from build123d import *

# Parameters (mm, degrees)
SKETCH_1_W          = 95
SKETCH_1_H          = 40
SKETCH_1_R          = 2.025
EXTRUDE_1_DEPTH     = 4
FILLET_1_R          = 4.5
SKETCH_2_W          = 79
SKETCH_2_H          = 24
CUT_EXTRUDE_1_DEPTH = 10
FILLET_2_R          = 3
SKETCH_3_R          = 2.025
CUT_EXTRUDE_2_DEPTH = 10
SKETCH_4_R          = 6
SKETCH_4_R_2        = 2.025
EXTRUDE_2_DEPTH     = 4
FILLET_3_R          = 5


with BuildPart() as part:
    # 草图1 → 凸台-拉伸1 (new body)
    with BuildSketch(Plane.XY):
        Rectangle(SKETCH_1_W, SKETCH_1_H)
        with Locations((-42, -14.5)):
            Circle(SKETCH_1_R, mode=Mode.SUBTRACT)
        with Locations((42, -14.5)):
            Circle(SKETCH_1_R, mode=Mode.SUBTRACT)
        with Locations((42, 14.5)):
            Circle(SKETCH_1_R, mode=Mode.SUBTRACT)
        with Locations((-42, 14.5)):
            Circle(SKETCH_1_R, mode=Mode.SUBTRACT)
        with BuildLine():
            Line((47.5, -20), (-47.5, -20))
            Line((-47.5, -20), (-47.5, -25))
            Line((-47.5, -25), (-117.089181798, -94.947092696))
            ThreePointArc((-117.089181798, -94.947092696), (-113.838679914, -92.766120181), (-110, -92))
            Line((-110, -92), (110, -92))
            ThreePointArc((110, -92), (113.838679914, -92.766120181), (117.089181798, -94.947092696))
            Line((117.089181798, -94.947092696), (47.5, -25))
            Line((47.5, -25), (47.5, -20))
        make_face()
        with BuildLine():
            Line((110, -92), (-110, -92))
            ThreePointArc((-110, -92), (-120, -102), (-110, -112))
            Line((-110, -112), (110, -112))
            ThreePointArc((110, -112), (120, -102), (110, -92))
        make_face()
        with Locations((110, -102)):
            Circle(SKETCH_1_R, mode=Mode.SUBTRACT)
        with Locations((55, -102)):
            Circle(SKETCH_1_R, mode=Mode.SUBTRACT)
        with Locations((0, -102)):
            Circle(SKETCH_1_R, mode=Mode.SUBTRACT)
        with Locations((-55, -102)):
            Circle(SKETCH_1_R, mode=Mode.SUBTRACT)
        with Locations((-110, -102)):
            Circle(SKETCH_1_R, mode=Mode.SUBTRACT)
    extrude(amount=EXTRUDE_1_DEPTH)

    # 圆角1
    fillet_1_edges = [part.edges().sort_by_distance(p)[0] for p in [
        (-47.5, -25, 2),
        (-47.5, 20, 2),
        (47.5, 20, 2),
        (47.5, -25, 2),
    ]]
    fillet(fillet_1_edges, radius=FILLET_1_R)

    # 草图2 → 切除-拉伸1 (cut)
    with BuildSketch(Plane.XY.offset(4)):
        Rectangle(SKETCH_2_W, SKETCH_2_H)
        Polygon((-39.5, -84.228054643), (-39.5, -20), (-4, -20), (-4, -55), align=None)
        Polygon((4, -55), (39.5, -84.228054643), (39.5, -20), (4, -20), align=None)
        Polygon((39.5, -92), (0, -59.478643425), (0, -92), align=None)
        Polygon((0, -92), (0, -59.478643425), (-39.5, -92), align=None)
        Polygon((51.5, -92), (51.5, -38.945557904), (104.282968869, -92), align=None)
        Polygon((-104.282968869, -92), (-51.5, -92), (-51.5, -38.945557904), align=None)
        with BuildLine():
            Line((-100, -106), (-65, -106))
            ThreePointArc((-65, -106), (-61, -102), (-65, -98))
            Line((-65, -98), (-100, -98))
            ThreePointArc((-100, -98), (-104, -102), (-100, -106))
        make_face()
        with BuildLine():
            Line((-45, -106), (-10, -106))
            ThreePointArc((-10, -106), (-6, -102), (-10, -98))
            Line((-10, -98), (-45, -98))
            ThreePointArc((-45, -98), (-49, -102), (-45, -106))
        make_face()
        with BuildLine():
            Line((10, -106), (45, -106))
            ThreePointArc((45, -106), (49, -102), (45, -98))
            Line((45, -98), (10, -98))
            ThreePointArc((10, -98), (6, -102), (10, -106))
        make_face()
        with BuildLine():
            Line((65, -106), (100, -106))
            ThreePointArc((100, -106), (104, -102), (100, -98))
            Line((100, -98), (65, -98))
            ThreePointArc((65, -98), (61, -102), (65, -106))
        make_face()
    extrude(amount=-CUT_EXTRUDE_1_DEPTH, mode=Mode.SUBTRACT)

    # 圆角2
    fillet_2_edges = [part.edges().sort_by_distance(p)[0] for p in [
        (39.5, -12, 2),
        (-39.5, -12, 2),
        (-39.5, 12, 2),
        (39.5, 12, 2),
        (51.5, -92, 2),
        (51.5, -38.945557904, 2),
        (104.282968869, -92, 2),
        (0, -59.478643425, 2),
        (39.5, -92, 2),
        (-39.5, -92, 2),
        (39.5, -84.228054643, 2),
        (4, -55, 2),
        (4, -20, 2),
        (39.5, -20, 2),
        (-39.5, -84.228054643, 2),
        (-39.5, -20, 2),
        (-4, -20, 2),
        (-4, -55, 2),
        (-51.5, -92, 2),
        (-104.282968869, -92, 2),
        (-51.5, -38.945557904, 2),
    ]]
    fillet(fillet_2_edges, radius=FILLET_2_R)

    # 草图3 → 切除-拉伸2 (cut)
    with BuildSketch(Plane.XY.offset(4)):
        with Locations((-47.5, -34.5)):
            Circle(SKETCH_3_R)
        with Locations((-47.5, -59.5)):
            Circle(SKETCH_3_R)
        with Locations((47.5, -34.5)):
            Circle(SKETCH_3_R)
        with Locations((47.5, -59.5)):
            Circle(SKETCH_3_R)
    extrude(amount=-CUT_EXTRUDE_2_DEPTH, mode=Mode.SUBTRACT)

    # 草图4 → 凸台-拉伸2 (add)
    with BuildSketch(Plane.XY.offset(4)):
        with Locations((-47.5, -59.5)):
            Circle(SKETCH_4_R)
        with Locations((-47.5, -59.5)):
            Circle(SKETCH_4_R_2, mode=Mode.SUBTRACT)
        with Locations((47.5, -59.5)):
            Circle(SKETCH_4_R)
        with Locations((47.5, -59.5)):
            Circle(SKETCH_4_R_2, mode=Mode.SUBTRACT)
    extrude(amount=-EXTRUDE_2_DEPTH)

    # 圆角3
    fillet_3_edges = [part.edges().sort_by_distance(p)[0] for p in [
        (-51.5, -63.972135955, 2),
        (-51.5, -55.027864045, 2),
        (51.5, -63.972135955, 2),
        (51.5, -55.027864045, 2),
    ]]
    fillet(fillet_3_edges, radius=FILLET_3_R)


solid = part.part
Part model, mm, in its own coordinate system. A direction names the side the tool comes from. Round coordinates to 2 decimals unless told otherwise and drop trailing zeros. Write each loop counter-clockwise with the first axis right and the second up, starting at its lowest first coordinate (ties: lowest second). Pieces come first, ordered by that corner, then holes. Notation, with made-up numbers: M 19,-31 L 30,-31 A17 cw 30,-17 Z; hole C 47.5,68.5 d2. An arc over 180 degrees is marked long. Return JSON: item names as keys, results as strings. Group by question number.
(1) Two-plate mould, pull along X, no slides. Class faces 3 (the face through (-46.217, 18.647, 2.028)), 4 (the face through (-1, -55, 4)), 5 (the face through (-77.61, -65.19, 2.03)), 6 (the face through (-17.26, -73.69, 2.03)): +X half, -X half, draft (parallel to the pull), parting line (faces both ways), or undercut.
(2) Saw through at A-A on y = 1. Write the cut outline in (x, z), then the cut area to 3 significant figures.
(3) Which spindle directions (+Z, -Z, +X, -X, +Y, -Y) get a long thin tool onto all of the face, cutting with end or side? Do faces 1 (the face through (19.637, -67.874, 2.028)), 2 (the face through (-82.47, -60.15, 1.97)). Say none if no direction does.
(4) Saw through at C-C on z = 2.9. Count the separate pieces of the cut face and the enclosed holes in it, then the cut area to 3 significant figures.
(5) Pin check, flat tips, straight feed: pin 1 Ø2 at (x, z) = (75, 3) entering from +Y; pin 2 Ø1.2 at (y, z) = (-4.5, 2.5) entering from -X; pin 3 Ø2 at (y, z) = (-51, 1.5) entering from +X. Stop position of each tip, or through.
(6) Drill centre lines: probe 1 along Y at (x, z) = (-42, 0.8) (3 decimals); probe 2 along Y at (x, z) = (0, 0.9) (3 decimals); probe 3 along Y at (x, z) = (-66, 1.8). Where is each one in solid material? Low to high.
(7) Saw through at B-B on x = -25. Write the cut outline in (y, z).
(8) Saw through at D-D on y = -69. Write the cut outline in (x, z), then the cut area to 3 significant figures.
Returned:
{
 "1": {"face 3": "-X half", "face 4": "draft", "face 5": "undercut", "face 6": "undercut"},
 "2": {"outline": "M -47.5,0 L -39.5,0 L -39.5,4 L -47.5,4 Z; M 39.5,0 L 47.5,0 L 47.5,4 L 39.5,4 Z", "area": "64.0 mm²"},
 "3": {"face 1": "+Z, -Z", "face 2": "+Z, -Z, -X, +Y"},
 "4": {"separate pieces": "1", "enclosed holes": "23", "area": "8,960 mm²"},
 "5": {"pin 1": "y = -51.64", "pin 2": "x = -47.5", "pin 3": "x = 74.36"},
 "6": {"probe 1": "-112 to -106, -98 to -16.525, -12.475 to 12.475, 16.525 to 20", "probe 2": "-112 to -104.025, -99.975 to -92, -60.365 to -12, 12 to 20", "probe 3": "-112 to -106, -98 to -92, -53.52 to -43.6"},
 "7": {"outline": "M -112,0 L -106,0 L -106,4 L -112,4 Z; M -98,0 L -92,0 L -92,4 L -98,4 Z; M -80.06,0 L -72.29,0 L -72.29,4 L -80.06,4 Z; M -20,0 L -12,0 L -12,4 L -20,4 Z; M 12,0 L 20,0 L 20,4 L 12,4 Z"},
 "8": {"outline": "M -91.27,0 L -81.4,0 L -81.4,4 L -91.27,4 Z; M -51.5,0 L -39.5,0 L -39.5,4 L -51.5,4 Z; M -21,0 L -11.56,0 L -11.56,4 L -21,4 Z; M 11.56,0 L 21,0 L 21,4 L 11.56,4 Z; M 39.5,0 L 51.5,0 L 51.5,4 L 39.5,4 Z; M 81.4,0 L 91.27,0 L 91.27,4 L 81.4,4 Z", "area": "251 mm²"}
}
